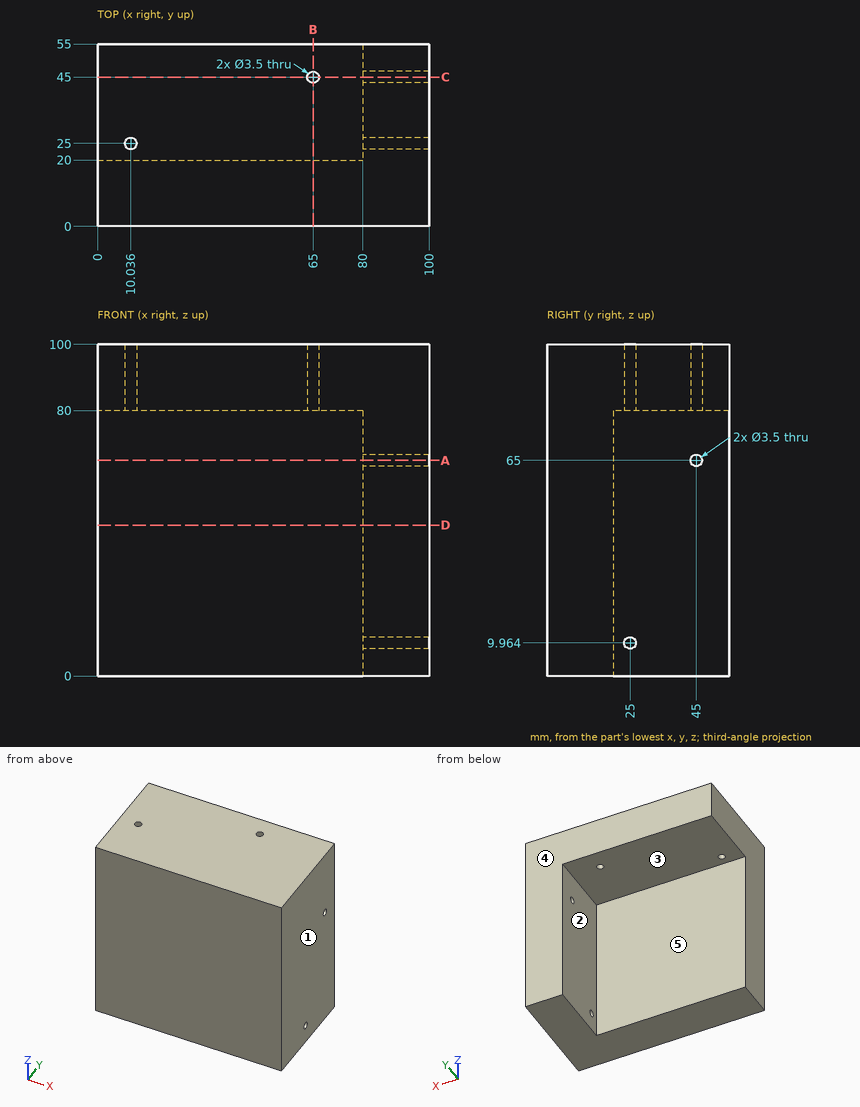
Design review of the part shown in the three views and the two pictorial views. Dimensions are in mm from the part's minimum x, y and z. A direction names the side the tool comes from. Coordinates: 2 decimals unless noted, no trailing zeros. Order: outer loops, then holes, each group sorted by start corner. A loop starts at its lowest first (then second) coordinate and runs counter-clockwise, first axis right, second up. Notation, with made-up numbers: (2.5, 46.5) - (45.5, 46.5) arc R31 ccw to (45.5, 77.5) - close; hole circle Ø5 at (-22.75, -10). An arc over 180 degrees is marked (long way). One line per question, with ' | ' between items.
Q1. Consider section D-D, the plane z = 45.5. Give the boundary of the cut face in (x, y).
Answer key:
outline: (0, 0) - (100, 0) - (100, 55) - (80, 55) - (80, 20) - (0, 20) - close
Q2. For the marked faces 4 and 5, list the 3-axis set-ups (+Z, -Z, +X, -X, +Y, -Y) from which the entire face can be reached by the end or side of a thin tool; tool diameter is ignored.
Answer key:
face 4: +Z, -Z, +X, -X, +Y | face 5: -Z, -X, +Y
Q3. Consider section B-B, the plane x = 65. Give the boundary of the cut face in (y, z), then the cut area to 3 significant figures.
Answer key:
outline: (0, 0) - (20, 0) - (20, 80) - (43.25, 80) - (43.25, 100) - (0, 100) - close; (46.75, 80) - (55, 80) - (55, 100) - (46.75, 100) - close | area: 2,630 mm2
Q4. Consider section C-C, the plane y = 45. Give the boundary of the cut face in (x, z), then the cut area to 3 significant figures.
Answer key:
outline: (0, 80) - (63.25, 80) - (63.25, 100) - (0, 100) - close; (66.75, 80) - (80, 80) - (80, 66.75) - (100, 66.75) - (100, 100) - (66.75, 100) - close; (80, 0) - (100, 0) - (100, 63.25) - (80, 63.25) - close | area: 3,460 mm2
Q5. Clearance check with flat-ended pins moving along their axes: pin 1 Ø6 at (y, z) = (29, 54) entering from -X; pin 2 Ø3 at (x, y) = (10.04, 25) entering from -Z; pin 3 Ø5 at (x, y) = (17, 43.5) entering from -Z. State where each tip first meets the part, or that it passes through.
Answer key:
pin 1: stops at x = 80 | pin 2: passes through | pin 3: stops at z = 80
Q6. The part is to be moulded in two halves that separate along X. For the marked faces 1, 2 and 3, say which applies: +X half, -X half, draft (parallel to the pull), parting line (faces both ways), or undercut.
Answer key:
face 1: +X half | face 2: -X half | face 3: draft
Q7. Consider section A-A, the plane z = 65. Give the boundary of the cut face in (x, y).
Answer key:
outline: (0, 0) - (100, 0) - (100, 43.25) - (80, 43.25) - (80, 20) - (0, 20) - close; (80, 46.75) - (100, 46.75) - (100, 55) - (80, 55) - close
Q8. To check wall thickness, follow line 1 along X through (y, z) = (45, 88.75); line 2 along Z through (x, y) = (95.5, 25). State the ranges of each line that lie inside material, in increasing order.
Answer key:
line 1: x = 0 to 63.25, 66.75 to 100 | line 2: z = 0 to 8.21, 11.71 to 100
